from build123d import *

# Parameters (mm, degrees)
SKETCH1_W           = 160.02
SKETCH1_H           = 127
BOSS_EXTRUDE2_DEPTH = 6.35
SKETCH2_R           = 3.175
CUT_EXTRUDE1_DEPTH  = 7.35
SKETCH8_R           = 2.286
CUT_EXTRUDE4_DEPTH  = 7.35
SKETCH10_R          = 4.826
SKETCH10_R_2        = 2.286
BOSS_EXTRUDE3_DEPTH = 3.81
BOSS_EXTRUDE4_DEPTH = 3.81
CHAMFER1_SIZE       = 2.54
CUT_EXTRUDE5_DEPTH  = 11.16


with BuildPart() as part:
    # Sketch1 → Boss-Extrude2 (new body)
    with BuildSketch(Plane(origin=(0, 0, 0), x_dir=(1, 0, 0), z_dir=(0, 1, 0))):
        with BuildLine():
            Line((0, 0), (0, 25.4))
            ThreePointArc((0, 25.4), (3.719743879, 34.380256121), (12.7, 38.1))
            Line((12.7, 38.1), (190.5, 38.1))
            ThreePointArc((190.5, 38.1), (199.480256121, 34.380256121), (203.2, 25.4))
            Line((203.2, 25.4), (203.2, -152.4))
            ThreePointArc((203.2, -152.4), (199.480256121, -161.380256121), (190.5, -165.1))
            Line((190.5, -165.1), (12.7, -165.1))
            ThreePointArc((12.7, -165.1), (3.719743879, -161.380256121), (0, -152.4))
            Line((0, -152.4), (0, -127))
            Line((0, -127), (0, 0))
        make_face()
        with Locations((101.6, -63.5)):
            Rectangle(SKETCH1_W, SKETCH1_H, mode=Mode.SUBTRACT)
    extrude(amount=BOSS_EXTRUDE2_DEPTH)

    # Sketch2 → Cut-Extrude1 (cut, through all)
    with BuildSketch(Plane(origin=(0, 6.35, 0), x_dir=(1, 0, 0), z_dir=(0, 1, 0))):
        with Locations((12.7, 25.4)):
            Circle(SKETCH2_R)
        with Locations((190.5, 25.4)):
            Circle(SKETCH2_R)
        with Locations((190.5, -152.4)):
            Circle(SKETCH2_R)
        with Locations((12.7, -152.4)):
            Circle(SKETCH2_R)
    extrude(amount=-CUT_EXTRUDE1_DEPTH, mode=Mode.SUBTRACT)

    # Sketch8 → Cut-Extrude4 (cut, through all)
    with BuildSketch(Plane(origin=(0, 0, 0), x_dir=(-1, 0, 0), z_dir=(0, -1, 0))):
        with Locations((-24.197781122, 13.902218878)):
            Circle(SKETCH8_R)
        with Locations((-24.197781122, -140.902218878)):
            Circle(SKETCH8_R)
        with Locations((-179.002218878, -140.902218878)):
            Circle(SKETCH8_R)
        with Locations((-179.002218878, 13.902218878)):
            Circle(SKETCH8_R)
    extrude(amount=-CUT_EXTRUDE4_DEPTH, mode=Mode.SUBTRACT)

    # Sketch10 → Boss-Extrude3 (add)
    with BuildSketch(Plane(origin=(0, 0, 0), x_dir=(-1, 0, 0), z_dir=(0, -1, 0))):
        with Locations((-44.45, 12.7)):
            Circle(SKETCH10_R)
        with Locations((-44.45, 12.7)):
            Circle(SKETCH10_R_2, mode=Mode.SUBTRACT)
        with Locations((-158.75, 12.7)):
            Circle(SKETCH10_R)
        with Locations((-158.75, 12.7)):
            Circle(SKETCH10_R_2, mode=Mode.SUBTRACT)
        with Locations((-158.75, -139.7)):
            Circle(SKETCH10_R)
        with Locations((-158.75, -139.7)):
            Circle(SKETCH10_R_2, mode=Mode.SUBTRACT)
        with Locations((-44.45, -139.7)):
            Circle(SKETCH10_R)
        with Locations((-44.45, -139.7)):
            Circle(SKETCH10_R_2, mode=Mode.SUBTRACT)
    extrude(amount=BOSS_EXTRUDE3_DEPTH)

    # Sketch11 → Boss-Extrude4 (add)
    with BuildSketch(Plane.XZ):
        with BuildLine():
            Line((174.07128, -38.1), (187.384850533, -24.786429467))
            ThreePointArc((187.384850533, -24.786429467), (187.552268433, -26.579620112), (188.668154157, -27.993253903))
            Line((188.668154157, -27.993253903), (178.561408061, -38.1))
            Line((178.561408061, -38.1), (174.07128, -38.1))
        make_face()
        with BuildLine():
            Line((203.2, -8.97128), (203.2, -13.461408061))
            Line((203.2, -13.461408061), (193.093253903, -23.568154157))
            ThreePointArc((193.093253903, -23.568154157), (191.679620112, -22.452268433), (189.886429467, -22.284850533))
            Line((189.886429467, -22.284850533), (203.2, -8.97128))
        make_face()
        with BuildLine():
            Line((10.106746097, -23.568154157), (0, -13.461408061))
            Line((0, -13.461408061), (0, -8.97128))
            Line((0, -8.97128), (13.313570533, -22.284850533))
            ThreePointArc((13.313570533, -22.284850533), (11.520379888, -22.452268433), (10.106746097, -23.568154157))
        make_face()
        with BuildLine():
            Line((15.815149467, -24.786429467), (29.12872, -38.1))
            Line((29.12872, -38.1), (24.638591939, -38.1))
            Line((24.638591939, -38.1), (14.531845843, -27.993253903))
            ThreePointArc((14.531845843, -27.993253903), (15.647731567, -26.579620112), (15.815149467, -24.786429467))
        make_face()
        with BuildLine():
            Line((14.531845843, 154.993253903), (24.638591939, 165.1))
            Line((24.638591939, 165.1), (29.12872, 165.1))
            Line((29.12872, 165.1), (15.815149467, 151.786429467))
            ThreePointArc((15.815149467, 151.786429467), (15.647731567, 153.579620112), (14.531845843, 154.993253903))
        make_face()
        with BuildLine():
            Line((13.313570533, 149.284850533), (0, 135.97128))
            Line((0, 135.97128), (0, 140.461408061))
            Line((0, 140.461408061), (10.106746097, 150.568154157))
            ThreePointArc((10.106746097, 150.568154157), (11.520379888, 149.452268433), (13.313570533, 149.284850533))
        make_face()
        with BuildLine():
            Line((193.093253903, 150.568154157), (203.2, 140.461408061))
            Line((203.2, 140.461408061), (203.2, 135.97128))
            Line((203.2, 135.97128), (189.886429467, 149.284850533))
            ThreePointArc((189.886429467, 149.284850533), (191.679620112, 149.452268433), (193.093253903, 150.568154157))
        make_face()
        with BuildLine():
            Line((187.384850533, 151.786429467), (174.07128, 165.1))
            Line((174.07128, 165.1), (178.561408061, 165.1))
            Line((178.561408061, 165.1), (188.668154157, 154.993253903))
            ThreePointArc((188.668154157, 154.993253903), (187.552268433, 153.579620112), (187.384850533, 151.786429467))
        make_face()
    extrude(amount=BOSS_EXTRUDE4_DEPTH)

    # Chamfer1
    chamfer1_edges = [part.edges().sort_by_distance(p)[0] for p in [
        (183.614781109, -3.81, -33.046626952),
        (198.146626952, -3.81, -18.514781109),
        (5.053373048, -3.81, -18.514781109),
        (19.585218891, -3.81, -33.046626952),
        (19.585218891, -3.81, 160.046626952),
        (5.053373048, -3.81, 145.514781109),
        (198.146626952, -3.81, 145.514781109),
        (183.614781109, -3.81, 160.046626952),
    ]]
    chamfer(chamfer1_edges, length=CHAMFER1_SIZE)

    # Sketch9 → Cut-Extrude5 (cut, through all)
    with BuildSketch(Plane(origin=(0, 6.35, 0), x_dir=(1, 0, 0), z_dir=(0, 1, 0))):
        Polygon((36.897781122, 0), (166.302218878, 0), (166.302218878, 7.62), (146.05, 7.62), (146.05, 16.51), (57.15, 16.51), (57.15, 7.62), (36.897781122, 7.62), align=None)
        Polygon((166.302218878, -127), (36.897781122, -127), (36.897781122, -134.62), (57.15, -134.62), (57.15, -143.51), (146.05, -143.51), (146.05, -134.62), (166.302218878, -134.62), align=None)
    extrude(amount=-CUT_EXTRUDE5_DEPTH, mode=Mode.SUBTRACT)


solid = part.part
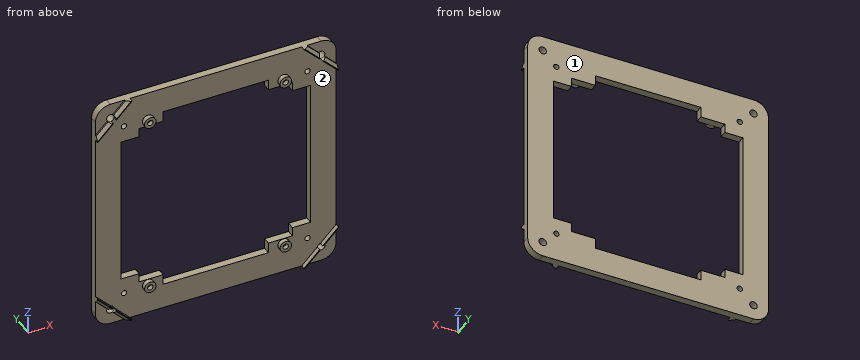
The model under review builds one solid part; all positions refer to its coordinate system, in mm. Face numbers are marked on the shaded views. Give positions to 0.01 mm unless a question says otherwise; leave off trailing zeros. Loops run counter-clockwise (first coordinate to the right, second up) from the corner with the lowest first, then second, coordinate; pieces in that order, holes last. Notation, with made-up numbers: (6.25, -17) -> (54.25, -17) arc R22 ccw to (54.25, 21) -> close; hole circle Ø9 at (-20.5, 43). An arc over 180 degrees is marked (long way). Answer as a JSON object with one key per item and string values. Group by question number.
Q1. Take a section at B-B (x = 117.5). Write out the cut boundary in (y, z), plus the area to 3 significant figures.
Q2. Draft analysis for pull direction X (two halves, no side actions). For the marked faces 1 and 2, state which applies: pulls with the +X half, pulls with the -X half, needs draft (parallel to the pull), parting line crosses it, or undercut.
Q3. Wall thickness on line 1 along X through (y, z) = (3.25, 152.4) (3 decimals); line 2 along Z through (x, y) = (190.5, 1.5) (3 decimals); line 3 along Z through (x, y) = (44.45, -1.85): over which ranges is each line inside the solid? List them lowest first.
Q4. Take a section at A-A (z = -3). Write out the cut boundary in (x, y).
Q5. Insertion check: pin 1 (7.5 mm diameter, centred on x = 17.5, z = 155, fed in from -Y); pin 2 (1.4 mm diameter, centred on x = 160, z = 139, fed in from -Y); pin 3 (2.5 mm diameter, centred on x = 24.2, z = -13.9, fed in from -Y). Each pin has a flat end and moves straight along its axis. Give the tip position at first contact, or say it passes through.
Q6. Take a section at C-C (y = 2). State how many separate pieces and enclosed holes the cut face has, plus the area to 3 significant figures.
Answer below:
{
 "1": {"outline": "(0, -38.1) -> (6.35, -38.1) -> (6.35, -16.51) -> (0, -16.51) -> close; (0, 143.51) -> (6.35, 143.51) -> (6.35, 165.1) -> (0, 165.1) -> close", "area": "274 mm2"},
 "2": {"face 1": "needs draft", "face 2": "undercut"},
 "3": {"line 1": "x = 0 to 9.525, 15.875 to 187.325, 193.675 to 203.2", "line 2": "z = -38.1 to -28.575, -22.225 to 149.225, 155.575 to 165.1", "line 3": "z = -17.53 to -14.99, -10.41 to -7.87, 134.87 to 137.41, 141.99 to 144.53"},
 "4": {"outline": "(0, 0) -> (36.9, 0) -> (36.9, 6.35) -> (0, 6.35) -> close; (166.3, 0) -> (203.2, 0) -> (203.2, 6.35) -> (166.3, 6.35) -> close"},
 "5": {"pin 1": "stops at y = -3.81", "pin 2": "stops at y = 0", "pin 3": "passes through"},
 "6": {"separate pieces": "1", "enclosed holes": "9", "area": "17,100 mm2"}
}
